from build123d import *

# Parameters (mm, degrees)
BOSS_EXTRU_1_DEPTH = 5


with BuildPart() as part:
    # Esquisse1 → Boss.-Extru.1 (new body)
    with BuildSketch(Plane(origin=(0, 0, 0), x_dir=(1, 0, 0), z_dir=(0, 1, 0))):
        with BuildLine():
            ThreePointArc((-88.017976153, -38.015428103), (-86.50201361, -41.562295618), (-84.458479206, -44.833744647))
            Line((-84.458479206, -44.833744647), (-81.815842439, -42.884303709))
            ThreePointArc((-81.815842439, -42.884303709), (-70.968463998, -15.424955777), (-43.384090899, -25.950342641))
            ThreePointArc((-43.384090899, -25.950342641), (-44.585088361, -5.046948778), (-31.398618719, 11.21685423))
            ThreePointArc((-31.398618719, 11.21685423), (-60.563222829, 19.936478121), (-50.379796194, 48.622777911))
            ThreePointArc((-50.379796194, 48.622777911), (-58.97592755, 46.948798531), (-66.46729281, 42.41281707))
            ThreePointArc((-66.46729281, 42.41281707), (-89.429119341, 5.46405326), (-88.017976153, -38.015428103))
        make_face()
    extrude(amount=BOSS_EXTRU_1_DEPTH)


solid = part.part
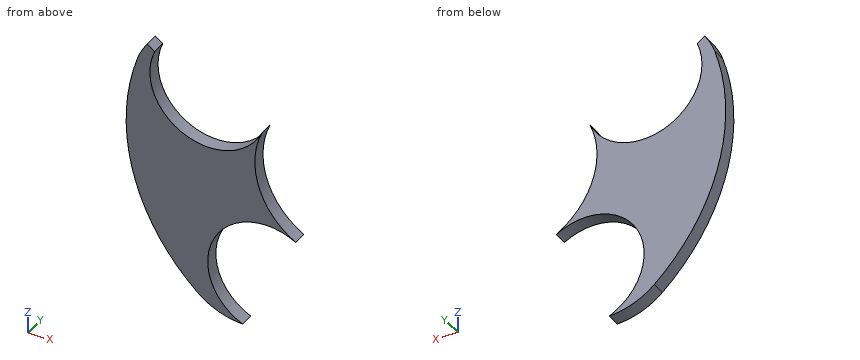
Geometry: final body of the model. Coordinates: model frame, mm. Give positions to 0.01 mm unless a question says otherwise; leave off trailing zeros. Loops run counter-clockwise (first coordinate to the right, second up) from the corner with the lowest first, then second, coordinate; pieces in that order, holes last. Notation, with made-up numbers: M 65,-10 L 98,-10 A11 cw 98,7 Z; hole C -38,58 d8. An arc over 180 degrees is marked long. Put each result on its own line as item: value. Start each with the question number.
1) Cut plane C-C (z = 21). Output: boundary loops of the cut face in (x, y), then the cut area to 3 significant figures.
2) Cut plane D-D (z = 8.5). Output: boundary loops of the cut face in (x, y).
3) Cut plane A-A (x = -53). Output: boundary loops of the cut face in (y, z).
4) Ray query, line 1 along X through (y, z) = (4.3, 23); line 2 along Z through (x, y) = (-58, 4.55); line 3 along Z through (x, y) = (-49, 4.5). Return the intervals inside material, ascending.
5) Contact query for flat-ended pins moving along their axis: pin 1 (8 mm diameter, centred on x = -76, z = 32, fed in from -Y); pin 2 (1.5 mm diameter, centred on y = 2, z = 6, fed in from -X). Output: stop coordinate, or through.
Verdict:
1. outline: M -91.65,0 L -78.47,0 L -78.47,5 L -91.65,5 Z; M -46.54,0 L -45.11,0 L -45.11,5 L -46.54,5 Z
1. area: 73.0 mm2
2. outline: M -91.79,0 L -45.47,0 L -45.47,5 L -91.79,5 Z
3. outline: M 0,-48.44 L 5,-48.44 L 5,-47.23 L 0,-47.23 Z; M 0,-11.65 L 5,-11.65 L 5,15.91 L 0,15.91 Z
4. line 1: -91.44 to -79.98, -45.02 to -44.54
4. line 2: -47.3 to -42.85, -16.03 to 14.13
4. line 3: -9.7 to 18.56
5. pin 1: through
5. pin 2: x = -91.64
